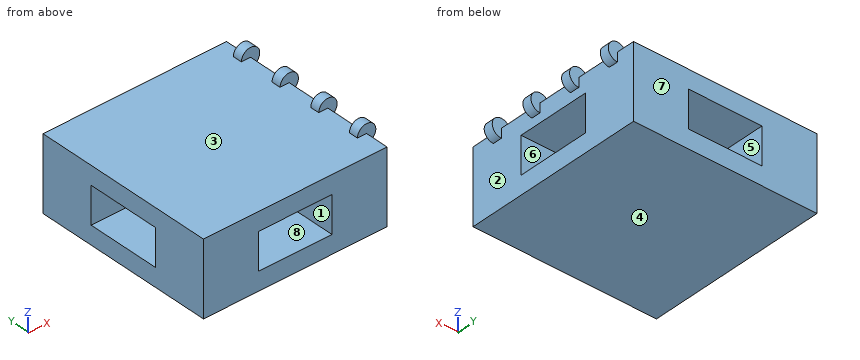
```python
from build123d import *

# Parameters (mm, degrees)
F0_W     = 100
F0_H     = 100
F1_DEPTH = 10
F2_W     = 30
F2_H     = 30
F3_DEPTH = 20
F5_W     = 100
F5_H     = 100
F6_DEPTH = 10
F7_W     = 5
F7_H     = 5


with BuildPart() as f1:
    # F0 (on Top) → F1 (new body)
    with BuildSketch(Plane.XY):
        Rectangle(F0_W, F0_H)
    extrude(amount=F1_DEPTH)

    # F2 (on face) → F3 (join)
    with BuildSketch(Plane.XY.offset(10)):
        with Locations((-35, 35)):
            Rectangle(F2_W, F2_H)
        with Locations((35, 35)):
            Rectangle(F2_W, F2_H)
        with Locations((-35, -35)):
            Rectangle(F2_W, F2_H)
        with Locations((35, -35)):
            Rectangle(F2_W, F2_H)
    extrude(amount=F3_DEPTH)

    # F5 (on offset) → F6 (join)
    with BuildSketch(Plane.XY.offset(30)):
        Rectangle(F5_W, F5_H)
    extrude(amount=F6_DEPTH)

    # F7 (on face) → F8 (revolve)
    with BuildSketch(Plane.XY.offset(40)):
        with Locations((47.5, 37.5)):
            Rectangle(F7_W, F7_H)
        with Locations((47.5, 13.3981328524)):
            Rectangle(F7_W, F7_H)
        with Locations((47.5, -10.7037342952)):
            Rectangle(F7_W, F7_H)
        with Locations((47.5, -34.8056014428)):
            Rectangle(F7_W, F7_H)
    revolve(axis=Axis((50, 0, 40), (0, -1, 0)))


solid = f1.part
```
Can you work these out from the model? Positions are in its coordinate system, mm. Face numbers are marked on the shaded views. A direction names the side the tool comes from. Give positions to 0.01 mm unless a question says otherwise; leave off trailing zeros. Order: outer loops, then holes, each group sorted by start corner. A loop starts at its lowest first (then second) coordinate and runs counter-clockwise, first axis right, second up. Notation, with made-up numbers: M -23,14.25 L -8,14.25 A29 cw -8,42.25 Z; hole C 32,-3.75 d9. An arc over 180 degrees is marked long. Write item = value, one per line. Start each with the question number.
Q1. Will these pins go through, and if not, where does the flat tip stop? pin 1 Ø2 at (y, z) = (-1, 33) entering from +X; pin 2 Ø8 at (x, y) = (-10, 18) entering from +Z.
Q2. I need wall thicknesses on probe 1 along Y at (x, z) = (29, 23.5); probe 2 along Z at (x, y) = (30.5, 8). Which ranges of each line are inside material? Lowest first, please. Write a range as [from, to].
Q3. Suppose I cut it at C-C (x = -42.5). Write out the boundary of the cut face in (y, z).
Q4. Suppose I cut it at A-A (z = 25). Write out the boundary of the cut face in (x, y), plus the area to 3 significant figures.
Q5. For the marked faces 4, 5, 6, 7 and 8, which set-ups out of +Z, -Z, +X, -X, +Y, -Y let a thin tool reach every point of the face, with its end or its side?
Q6. We'd pull the mould along X, two halves only. Please class the marked faces 1, 2 and 3: pulls with the +X half, pulls with the -X half, needs draft (parallel to the pull), parting line crosses it, or undercut.
Q7. Suppose I cut it at B-B (y = 13). Write out the boundary of the cut face in (x, z), plus the area to 3 significant figures.
Check result:
q1.pin_1 = 50
q1.pin_2 = 40
q2.probe_1 = [-50, -20], [20, 50]
q2.probe_2 = [0, 10], [30, 40]
q3.outline = M -50,0 L 50,0 L 50,40 L -50,40 Z; hole M -20,10 L 20,10 L 20,30 L -20,30 Z
q4.outline = M -50,-50 L -20,-50 L -20,-20 L -50,-20 Z; M -50,20 L -20,20 L -20,50 L -50,50 Z; M 20,-50 L 50,-50 L 50,-20 L 20,-20 Z; M 20,20 L 50,20 L 50,50 L 20,50 Z
q4.area = 3,600 mm2
q5.face_4 = -Z, +X, -X, +Y, -Y
q5.face_5 = +Y, -Y
q5.face_6 = +X, -X
q5.face_7 = +Z, -Z, +X, -X, +Y
q5.face_8 = none
q6.face_1 = undercut
q6.face_2 = pulls with the +X half
q6.face_3 = needs draft
q7.outline = M -50,0 L 50,0 L 50,10 L -50,10 Z; M -50,30 L 50,30 L 50,35 A5 ccw long 45,40 L -50,40 Z
q7.area = 2,060 mm2
